Read the model definition and answer for the solid it produces. Units are mm, in the model's axes. Coordinates: 2 decimals unless noted, no trailing zeros. Loops run counter-clockwise (first coordinate to the right, second up) from the corner with the lowest first, then second, coordinate; pieces in that order, holes last. Notation, with made-up numbers: (35, 36.25) -> (66, 36.25) arc R19 ccw to (66, 71.25) -> close; hole circle Ø9 at (-10.5, 77.5). An arc over 180 degrees is marked (long way). Answer in a Markdown table with one row per item.
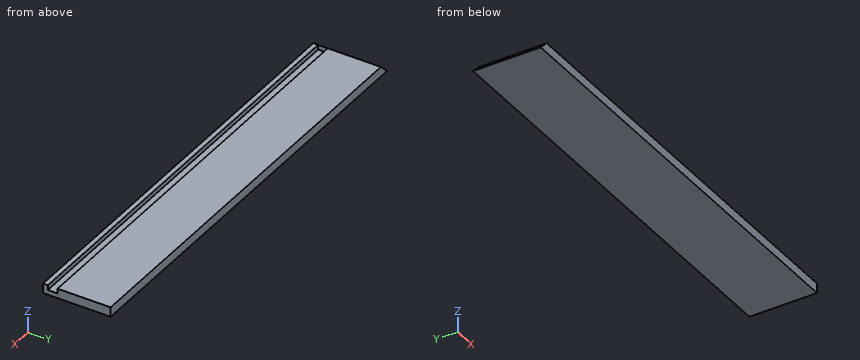
```python
from build123d import *

# Parameters (mm, degrees)
SKETCH1_W           = 577.85
SKETCH1_H           = 88.9
BOSS_EXTRUDE1_DEPTH = 12.7
CUT_EXTRUDE1_DEPTH  = 89.9
SKETCH4_W           = 565.15
SKETCH4_H           = 12.7
CUT_EXTRUDE3_DEPTH  = 6.35


with BuildPart() as part:
    # Sketch1 → Boss-Extrude1 (new body)
    with BuildSketch(Plane.XY):
        with Locations((75.280996393, 74.68264202)):
            Rectangle(SKETCH1_W, SKETCH1_H)
    extrude(amount=BOSS_EXTRUDE1_DEPTH)

    # Sketch2 → Cut-Extrude1 (cut, through all)
    with BuildSketch(Plane(origin=(0, 119.13264202, 0), x_dir=(1, 0, 0), z_dir=(0, 1, 0))):
        Polygon((-200.944003607, -12.7), (-213.644003607, 0), (-213.644003607, -12.7), align=None)
    extrude(amount=-CUT_EXTRUDE1_DEPTH, mode=Mode.SUBTRACT)

    # Sketch4 → Cut-Extrude3 (cut)
    with BuildSketch(Plane.XY.offset(12.7)):
        with Locations((81.630996393, 42.93264202)):
            Rectangle(SKETCH4_W, SKETCH4_H)
    extrude(amount=-CUT_EXTRUDE3_DEPTH, mode=Mode.SUBTRACT)


solid = part.part
```
1. Given pin 1 Ø1.9 at (y, z) = (44, 10.5) entering from +X; pin 2 Ø4 at (x, y) = (130.5, 41) entering from +Z; pin 3 Ø12 at (x, y) = (25, 99.5) entering from -Z, each flat-ended and moving along its own axis, determine where each tip first touches the part or whether it passes through.
A:
| item | result |
|---|---|
| pin 1 | stops at x = -200.94 |
| pin 2 | stops at z = 6.35 |
| pin 3 | stops at z = 0 |
2. Find the intervals of material crossed by probe 1 along Y at (x, z) = (-159, 11.5); probe 2 along Z at (x, y) = (-49, 44.5); probe 3 along X at (y, z) = (58, 11), in increasing order.
A:
| item | result |
|---|---|
| probe 1 | y = 30.23 to 36.58, 49.28 to 119.13 |
| probe 2 | z = 0 to 6.35 |
| probe 3 | x = -202.64 to 364.21 |
3. A cutting plane is placed at B-B on z = 9.5. Give the vertices of the cut face in (x, y), and give its area (3 significant figures).
A:
| item | result |
|---|---|
| outline | (-204.14, 30.23) -> (364.21, 30.23) -> (364.21, 36.58) -> (-200.94, 36.58) -> (-200.94, 49.28) -> (364.21, 49.28) -> (364.21, 119.13) -> (-204.14, 119.13) -> close |
| area | 43,300 mm2 |
4. A cutting plane is placed at A-A on x = -15. Give the vertices of the cut face in (y, z).
A:
| item | result |
|---|---|
| outline | (30.23, 0) -> (119.13, 0) -> (119.13, 12.7) -> (49.28, 12.7) -> (49.28, 6.35) -> (36.58, 6.35) -> (36.58, 12.7) -> (30.23, 12.7) -> close |
